```python
from build123d import *

# Parameters (mm, degrees)
BOSS_EXTRUDE1_DEPTH      = 8.89
CUT_EXTRUDE6_DEPTH       = 112.74556725
CUT_EXTRUDE6_DEPTH_BACK  = 112.74556725
SKETCH9_R                = 1.267511842
SKETCH9_W                = 3.81
SKETCH9_H                = 8.128
SKETCH9_W_2              = 3.556
SKETCH9_H_2              = 13.97
SKETCH9_W_3              = 8.73125
SKETCH9_H_3              = 3.96875
CUT_EXTRUDE7_DEPTH       = 7.9375
CUT_EXTRUDE7_DEPTH_BACK  = 112.74556725
SKETCH4_W                = 34.29
SKETCH4_H                = 30.48
CUT_EXTRUDE8_DEPTH       = 112.74556725
CUT_EXTRUDE8_DEPTH_BACK  = 112.74556725
SKETCH3_R                = 5.08
CUT_EXTRUDE9_DEPTH       = 112.74556725
CUT_EXTRUDE9_DEPTH_BACK  = 112.74556725
SKETCH12_R               = 1.27
CUT_EXTRUDE10_DEPTH      = 112.74556725
CUT_EXTRUDE10_DEPTH_BACK = 112.74556725
SKETCH15_R               = 1.27
CUT_EXTRUDE11_DEPTH      = 112.74556725
CUT_EXTRUDE11_DEPTH_BACK = 112.74556725
SKETCH16_W               = 3.81
SKETCH16_H               = 11.43


with BuildPart() as part:
    # Sketch1 → Boss-Extrude1 (new body)
    with BuildSketch(Plane.XY):
        with BuildLine():
            Line((-3.314058103, 6.35), (48.26, 6.35))
            ThreePointArc((48.26, 6.35), (51.852102448, 4.862102448), (53.34, 1.27))
            Line((53.34, 1.27), (53.34, -92.71))
            ThreePointArc((53.34, -92.71), (51.852102448, -96.302102448), (48.26, -97.79))
            Line((48.26, -97.79), (16.846989059, -97.79))
            ThreePointArc((16.846989059, -97.79), (15.638688158, -97.644208035), (14.499741809, -97.215200367))
            Line((14.499741809, -97.215200367), (-16.7505185, -80.933552139))
            ThreePointArc((-16.7505185, -80.933552139), (-18.059258376, -79.955412607), (-18.989802686, -78.61241436))
            Line((-18.989802686, -78.61241436), (-28.309569459, -59.040904135))
            ThreePointArc((-28.309569459, -59.040904135), (-28.795802898, -57.127870198), (-28.51617555, -55.173917704))
            Line((-28.51617555, -55.173917704), (-8.107195629, 2.952923842))
            ThreePointArc((-8.107195629, 2.952923842), (-6.251501454, 5.414614163), (-3.314058103, 6.35))
        make_face()
    extrude(amount=BOSS_EXTRUDE1_DEPTH)

    # Sketch9 → Cut-Extrude6 (cut, two sides: drawn at the far end of the back side and taken through both)
    with BuildSketch(Plane(origin=(0, 0, 0), x_dir=(-1, 0, 0), z_dir=(0, 0, -1)).offset(-CUT_EXTRUDE6_DEPTH_BACK)):
        with Locations((-5.348417946, -30.953529248)):
            Circle(SKETCH9_R)
        with Locations((-32.218986844, -9.676052932)):
            Circle(SKETCH9_R)
        with Locations((-12.150498686, -12.37729109)):
            Circle(SKETCH9_R)
        with Locations((-12.150498686, -26.66479109)):
            Circle(SKETCH9_R)
        with Locations((-28.057248686, -12.37729109)):
            Circle(SKETCH9_R)
        with Locations((-5.348417946, -9.676052932)):
            Circle(SKETCH9_R)
        with Locations((-32.218986844, -30.953529248)):
            Circle(SKETCH9_R)
        with Locations((-28.057248686, -26.66479109)):
            Circle(SKETCH9_R)
        with Locations((-10.245904396, -20.31479109)):
            Rectangle(SKETCH9_W, SKETCH9_H)
        Polygon((-15.064842187, -33.01479109), (-23.802748686, -33.01479109), (-23.802748686, -26.66479109), (-20.913498686, -26.66479109), (-15.064842187, -26.66479109), align=None)
        with Locations((-35.010498686, -19.798068783)):
            Rectangle(SKETCH9_W_2, SKETCH9_H_2)
        with Locations((-19.310123686, -9.59916609)):
            Rectangle(SKETCH9_W_3, SKETCH9_H_3)
    extrude(amount=CUT_EXTRUDE6_DEPTH + CUT_EXTRUDE6_DEPTH_BACK, mode=Mode.SUBTRACT)

    # Sketch4 → Cut-Extrude7 (cut, two sides: drawn at the far end of the back side and taken through both)
    with BuildSketch(Plane.XY.offset(-CUT_EXTRUDE7_DEPTH_BACK)):
        with Locations((20.024498686, -18.415)):
            Rectangle(SKETCH4_W, SKETCH4_H)
    extrude(amount=CUT_EXTRUDE7_DEPTH + CUT_EXTRUDE7_DEPTH_BACK, mode=Mode.SUBTRACT)

    # Sketch3 → Cut-Extrude8 (cut, two sides: drawn at the far end of the back side and taken through both)
    with BuildSketch(Plane.XY.offset(8.89).offset(-CUT_EXTRUDE8_DEPTH_BACK)):
        with Locations(Location((3.878385852, -38.1, 0), (0, 0, 61.044975628))):
            Circle(SKETCH3_R)
        with Locations((-5.011614148, -46.99)):
            Circle(SKETCH3_R)
        with Locations((3.878385852, -55.88)):
            Circle(SKETCH3_R)
        with Locations((12.768385852, -46.99)):
            Circle(SKETCH3_R)
        with Locations((-9.144, -65.024)):
            Circle(SKETCH3_R)
        with Locations((3.048, -70.612)):
            Circle(SKETCH3_R)
        with Locations((15.24, -76.2)):
            Circle(SKETCH3_R)
    extrude(amount=CUT_EXTRUDE8_DEPTH + CUT_EXTRUDE8_DEPTH_BACK, mode=Mode.SUBTRACT)

    # Sketch12 → Cut-Extrude9 (cut, two sides: drawn at the far end of the back side and taken through both)
    with BuildSketch(Plane(origin=(0, 0, 0), x_dir=(-1, 0, 0), z_dir=(0, 0, -1)).offset(-CUT_EXTRUDE9_DEPTH_BACK)):
        with Locations((-48.0822, 2.286)):
            Circle(SKETCH12_R)
        with Locations((3.718687848, 1.651)):
            Circle(SKETCH12_R)
        with Locations((25.012261453, -59.761967182)):
            Circle(SKETCH12_R)
    extrude(amount=CUT_EXTRUDE9_DEPTH + CUT_EXTRUDE9_DEPTH_BACK, mode=Mode.SUBTRACT)

    # Sketch15 → Cut-Extrude10 (cut, two sides: drawn at the far end of the back side and taken through both)
    with BuildSketch(Plane(origin=(0, 0, 0), x_dir=(-1, 0, 0), z_dir=(0, 0, -1)).offset(-CUT_EXTRUDE10_DEPTH_BACK)):
        with Locations((18.034, -57.15)):
            Circle(SKETCH15_R)
        with Locations((-43.942, -85.852)):
            Circle(SKETCH15_R)
    extrude(amount=CUT_EXTRUDE10_DEPTH + CUT_EXTRUDE10_DEPTH_BACK, mode=Mode.SUBTRACT)

    # Sketch16 → Cut-Extrude11 (cut, two sides: drawn at the far end of the back side and taken through both)
    with BuildSketch(Plane(origin=(0, 0, 0), x_dir=(-1, 0, 0), z_dir=(0, 0, -1)).offset(-CUT_EXTRUDE11_DEPTH_BACK)):
        with Locations((-23.749, -79.121)):
            Rectangle(SKETCH16_W, SKETCH16_H)
        with Locations((-31.623, -79.121)):
            Rectangle(SKETCH16_W, SKETCH16_H)
    extrude(amount=CUT_EXTRUDE11_DEPTH + CUT_EXTRUDE11_DEPTH_BACK, mode=Mode.SUBTRACT)


solid = part.part
```
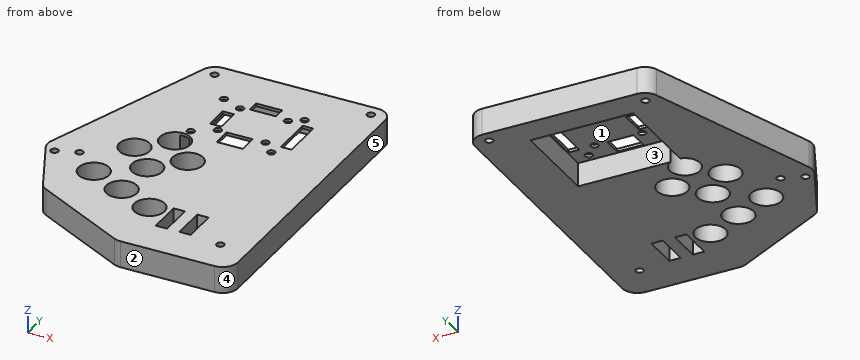
The model under review builds one solid part; all positions refer to its coordinate system, in mm. Face numbers are marked on the shaded views. A direction names the side the tool comes from. Give positions to 0.01 mm unless a question says otherwise; leave off trailing zeros. Write each loop counter-clockwise with the first axis right and the second up, starting at its lowest first coordinate (ties: lowest second). Pieces come first, ordered by that corner, then holes. Notation, with made-up numbers: M 88.25,-13 L 141.25,-13 A31 ccw 141.25,12 Z; hole C 61.25,-1.5 d1. An arc over 180 degrees is marked long. Answer in a Markdown table with one row per item.
Item 1: Add section A-A on y = -15. Give the boundary of the cut face in (x, z), plus the area to 3 significant figures.
Check sheet entries:
| item | result |
|---|---|
| outline | M -14.41,0 L 2.88,0 L 2.88,7.94 L 33.23,7.94 L 33.23,8.89 L -14.41,8.89 Z; M 36.79,7.94 L 37.17,7.94 L 37.17,0 L 53.34,0 L 53.34,8.89 L 36.79,8.89 Z |
| area | 327 mm2 |
Item 2: For line 1 along Y through (x, z) = (33, 5.25) (3 decimals); line 2 along X through (y, z) = (-83, 1.75); line 3 along X through (y, z) = (-59.5, 8), list the stretches that pass through material, from the lowest coordinate up.
Check sheet entries:
| item | result |
|---|---|
| line 1 | -97.79 to -84.836, -73.406 to -33.655, -3.175 to 6.35 |
| line 2 | -12.78 to 21.84, 25.65 to 29.72, 33.53 to 53.34 |
| line 3 | -28.09 to -26.25, -23.77 to 0.31, 7.44 to 53.34 |
Item 3: Add section D-D on z = 3.25. State how many separate pieces and enclosed holes the cut face has, plus the area to 3 significant figures.
Check sheet entries:
| item | result |
|---|---|
| separate pieces | 1 |
| enclosed holes | 14 |
| area | 5,530 mm2 |
Item 4: Tool access review of the marked faces 1 and 2: name each direction out of +Z, -Z, +X, -X, +Y, -Y from which nothing blocks a thin tool from reaching the whole face with its end or side.
Check sheet entries:
| item | result |
|---|---|
| face 1 | -Z |
| face 2 | +Z, -Z, +X, -X, -Y |
Item 5: Add section C-C on y = -57.15. Give the boundary of the cut face in (x, z).
Check sheet entries:
| item | result |
|---|---|
| outline | M -28.79,0 L -19.3,0 L -19.3,8.89 L -28.79,8.89 Z; M -16.76,0 L -1.04,0 L -1.04,8.89 L -16.76,8.89 Z; M 8.8,0 L 53.34,0 L 53.34,8.89 L 8.8,8.89 Z |
Item 6: Draft analysis for pull direction Y (two halves, no side actions). For the marked faces 3, 4 and 5, state which applies: +Y half, -Y half, draft (parallel to the pull), parting line (faces both ways), or undercut.
Check sheet entries:
| item | result |
|---|---|
| face 3 | undercut |
| face 4 | -Y half |
| face 5 | draft |
Item 7: For P1, Ø3, axis at x = 6.5, z = 3, coming from the -Y side; P2, Ø2, axis at y = -17, z = 5.5, coming from the -X side; P3, Ø2.5, axis at y = -81, z = 3, coming from the -X side, all flat-tipped, find the tip position at first contact; note any pin that passes through.
Check sheet entries:
| item | result |
|---|---|
| P1 | y = -93.83 |
| P2 | x = -15.46 |
| P3 | x = -18.25 |
Item 8: Add section B-B on y = -74.5. Give the boundary of the cut face in (x, z), plus the area to 3 significant figures.
Check sheet entries:
| item | result |
|---|---|
| outline | M -20.95,0 L -0.22,0 L -0.22,8.89 L -20.95,8.89 Z; M 6.32,0 L 10.45,0 L 10.45,8.89 L 6.32,8.89 Z; M 20.03,0 L 21.84,0 L 21.84,8.89 L 20.03,8.89 Z; M 25.65,0 L 29.72,0 L 29.72,8.89 L 25.65,8.89 Z; M 33.53,0 L 53.34,0 L 53.34,8.89 L 33.53,8.89 Z |
| area | 449 mm2 |
